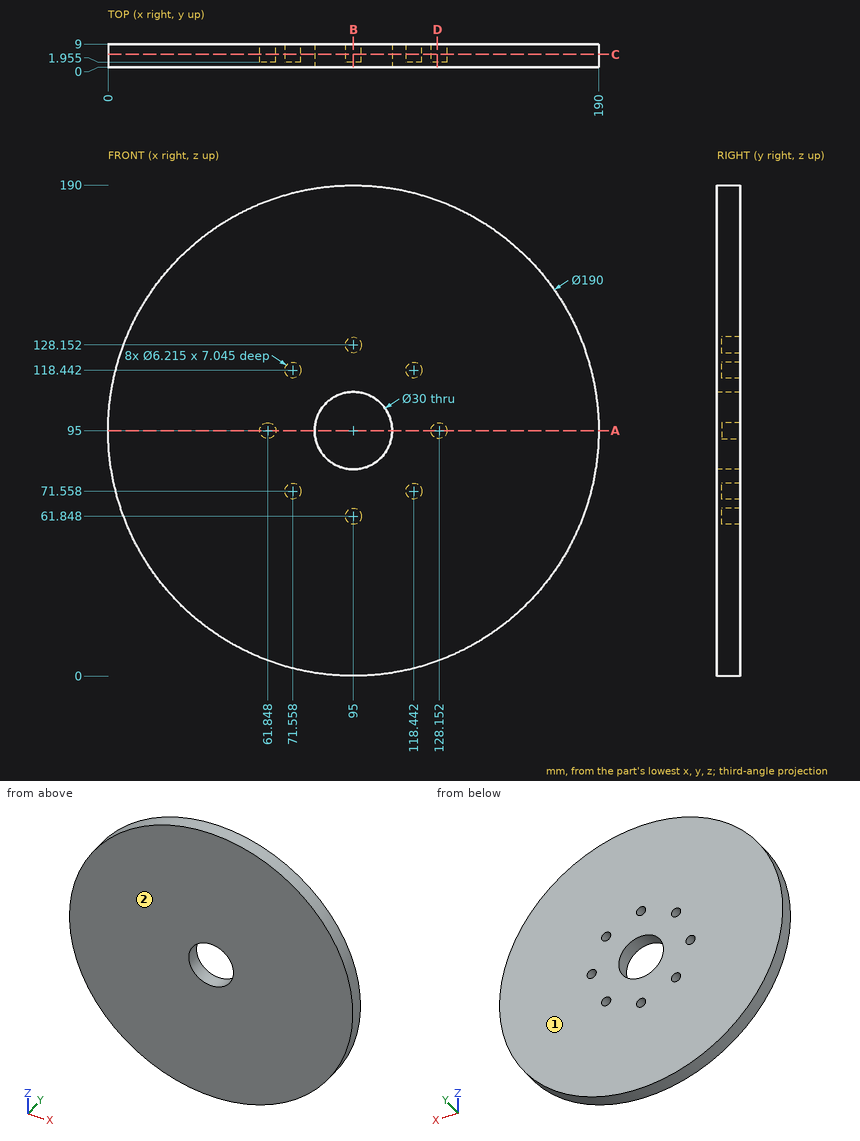
Design review of the part shown in the three views and the two pictorial views. Dimensions are in mm from the part's minimum x, y and z. Round coordinates to 2 decimals unless told otherwise and drop trailing zeros. Loops run counter-clockwise (first coordinate to the right, second up) from the corner with the lowest first, then second, coordinate; pieces in that order, holes last.
1) Consider section D-D on x = 127.5. State the section outline as (y, z) points (1 decimal), then the cut area to 3 significant figures.
Values follow:
outline: (0, 5.7) - (9, 5.7) - (9, 92) - (2, 92) - (2, 98) - (9, 98) - (9, 184.3) - (0, 184.3) - close
area: 1,560 mm2
2) Wall thickness on line 1 along X through (y, z) = (2.5, 95); line 2 along X through (y, z) = (4.5, 103); line 3 along X through (y, z) = (7.25, 118) (1 decimal): over which ranges is each line inside the solid? List them lowest first.
Values follow:
line 1: x = 0 to 58.74, 64.96 to 80, 110 to 125.04, 131.26 to 190
line 2: x = 0.34 to 82.31, 107.69 to 189.66
line 3: x = 2.8 to 68.5, 74.6 to 115.4, 121.5 to 187.2
3) Consider section B-B on x = 95. State the section outline as (y, z) points (1 decimal).
Values follow:
outline: (0, 0) - (9, 0) - (9, 58.7) - (2, 58.7) - (2, 65) - (9, 65) - (9, 80) - (0, 80) - close; (0, 110) - (9, 110) - (9, 125) - (2, 125) - (2, 131.3) - (9, 131.3) - (9, 190) - (0, 190) - close
4) Consider section C-C on y = 5. Give the number of separate pieces and of enclosed holes in the cut face, then the cut area to 3 significant figures.
Values follow:
separate pieces: 1
enclosed holes: 9
area: 27,400 mm2
5) Consider section A-A on z = 95. State the section outline as (x, y) points (1 decimal).
Values follow:
outline: (0, 0) - (80, 0) - (80, 9) - (65, 9) - (65, 2) - (58.7, 2) - (58.7, 9) - (0, 9) - close; (110, 0) - (190, 0) - (190, 9) - (131.3, 9) - (131.3, 2) - (125, 2) - (125, 9) - (110, 9) - close
6) Clearance check with flat-ended pins moving along their axes: P1, Ø5, axis at x = 128.15, z = 95, coming from the -Y side; P2, Ø5, axis at x = 118.44, z = 71.56, coming from the +Y side (1 decimal); P3, Ø4, axis at x = 151.5, y = 2, coming from the +Z side; P4, Ø5, axis at y = 2.5, z = 45.5, coming from the -X side. State where each tip first meets the part, or that it passes through.
Values follow:
P1: stops at y = 0
P2: stops at y = 2
P3: stops at z = 172.81
P4: stops at x = 12.44
7) The part is to be moulded in two halves that separate along Y. For the marked faces 1 and 2, say which applies: pulls with the +Y half, pulls with the -Y half, needs draft (parallel to the pull), parting line crosses it, or undercut.
Values follow:
face 1: pulls with the +Y half
face 2: pulls with the -Y half
